Design review of the part built by this model. Coordinates are the model's own, in mm. Give positions to 0.01 mm unless a question says otherwise; leave off trailing zeros. Write each loop counter-clockwise with the first axis right and the second up, starting at its lowest first coordinate (ties: lowest second). Pieces come first, ordered by that corner, then holes. Notation, with made-up numbers: M 42,18 L 59,18 A6 ccw 59,26 Z; hole C 26.5,-18.5 d1. An arc over 180 degrees is marked long. Use one line per item in the form item = value. Start each with the question number.
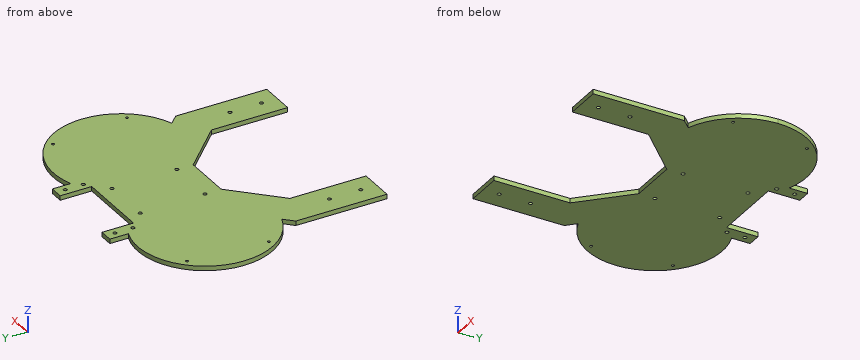
from build123d import *

# Parameters (mm, degrees)
SKETCH1_R           = 2
BOSS_EXTRUDE1_DEPTH = 5
SKETCH2_R           = 2
BOSS_EXTRUDE2_DEPTH = 5
BOSS_EXTRUDE3_START = -5
SKETCH3_R           = 1.4732
SKETCH3_R_2         = 2
BOSS_EXTRUDE3_DEPTH = 5


with BuildPart() as part:
    # Sketch1 → Boss-Extrude1 (new body)
    with BuildSketch(Plane.XY):
        Polygon((-40, 70), (-55, 70), (-55, -70), (55, -70), (55, 70), (40, 70), (40, 35), (-40, 35), align=None)
        with Locations((-27, -52)):
            Circle(SKETCH1_R, mode=Mode.SUBTRACT)
        with Locations((27, -52)):
            Circle(SKETCH1_R, mode=Mode.SUBTRACT)
        with Locations((-27, 20)):
            Circle(SKETCH1_R, mode=Mode.SUBTRACT)
        with Locations((-47.5, 40)):
            Circle(SKETCH1_R, mode=Mode.SUBTRACT)
        with Locations((-47.5, 60)):
            Circle(SKETCH1_R, mode=Mode.SUBTRACT)
        with Locations((27, 20)):
            Circle(SKETCH1_R, mode=Mode.SUBTRACT)
        with Locations((47.5, 40)):
            Circle(SKETCH1_R, mode=Mode.SUBTRACT)
        with Locations((47.5, 60)):
            Circle(SKETCH1_R, mode=Mode.SUBTRACT)
    extrude(amount=BOSS_EXTRUDE1_DEPTH)

    # Sketch2 → Boss-Extrude2 (add)
    with BuildSketch(Plane.XY):
        Polygon((-26.715726767, -70), (-55, -41.715726767), (-115, -101.715728753), (-115, -203), (-75, -203), (-75, -118.284271635), align=None)
        with Locations((-95, -185.5)):
            Circle(SKETCH2_R, mode=Mode.SUBTRACT)
        with Locations((-95, -150.5)):
            Circle(SKETCH2_R, mode=Mode.SUBTRACT)
    boss_extrude2 = extrude(amount=BOSS_EXTRUDE2_DEPTH)

    # Mirror1: Boss-Extrude2 across plane
    add(boss_extrude2.mirror(Plane(origin=(0, 0, 0), x_dir=(0, 0, 1), z_dir=(1, 0, 0))))

    # Sketch3 → Boss-Extrude3 (add)
    # profile 1 of 4: a face of its own
    with BuildSketch(Plane.XY.offset(5).offset(BOSS_EXTRUDE3_START)):
        with BuildLine():
            ThreePointArc((-55, 49.531907673), (-151.188193929, 4.063504127), (-105.126050476, -91.841778902))
            Line((-105.126050476, -91.841778902), (-55, -41.715726767))
            Line((-55, -41.715726767), (-55, 49.531907673))
        make_face()
        with Locations((-135.79276299, -59.716409454)):
            Circle(SKETCH3_R, mode=Mode.SUBTRACT)
        with Locations((-128.22970773, 26.72970773)):
            Circle(SKETCH3_R, mode=Mode.SUBTRACT)
    # profile 2 of 4: a face of its own
    with BuildSketch(Plane.XY.offset(5).offset(BOSS_EXTRUDE3_START)):
        with BuildLine():
            ThreePointArc((-105.126050476, -91.841778902), (-72.958779258, -95.619903442), (-42.197872056, -85.482144776))
            Line((-42.197872056, -85.482144776), (-26.715726767, -70))
            Line((-26.715726767, -70), (-23.719721734, -70))
            ThreePointArc((-23.719721734, -70), (-10.202344029, -47.138851639), (-5.5, -21))
            ThreePointArc((-5.5, -21), (-12.064844908, 9.685982916), (-30.610121267, 35))
            Line((-30.610121267, 35), (-40, 35))
            Line((-40, 35), (-40, 42.124876238))
            ThreePointArc((-40, 42.124876238), (-47.292831667, 46.247929123), (-55, 49.531907673))
            Line((-55, 49.531907673), (-55, -41.715726767))
            Line((-55, -41.715726767), (-105.126050476, -91.841778902))
        make_face()
        with Locations((-27, -52)):
            Circle(SKETCH3_R_2, mode=Mode.SUBTRACT)
        with Locations((-27, 20)):
            Circle(SKETCH3_R_2, mode=Mode.SUBTRACT)
        with Locations((-47.5, 40)):
            Circle(SKETCH3_R_2, mode=Mode.SUBTRACT)
    # profile 3 of 4: a face of its own
    with BuildSketch(Plane.XY.offset(5).offset(BOSS_EXTRUDE3_START)):
        with BuildLine():
            ThreePointArc((30.610121267, 35), (5.660968749, -16.088849276), (23.719721734, -70))
            Line((23.719721734, -70), (26.715726767, -70))
            Line((26.715726767, -70), (42.197872056, -85.482144776))
            ThreePointArc((42.197872056, -85.482144776), (72.958779258, -95.619903442), (105.126050476, -91.841778902))
            Line((105.126050476, -91.841778902), (55, -41.715726767))
            Line((55, -41.715726767), (55, 49.531907673))
            ThreePointArc((55, 49.531907673), (47.292831667, 46.247929123), (40, 42.124876238))
            Line((40, 42.124876238), (40, 35))
            Line((40, 35), (30.610121267, 35))
        make_face()
        with Locations((27, -52)):
            Circle(SKETCH3_R_2, mode=Mode.SUBTRACT)
        with Locations((27, 20)):
            Circle(SKETCH3_R_2, mode=Mode.SUBTRACT)
        with Locations((47.5, 40)):
            Circle(SKETCH3_R_2, mode=Mode.SUBTRACT)
    # profile 4 of 4: a face of its own
    with BuildSketch(Plane.XY.offset(5).offset(BOSS_EXTRUDE3_START)):
        with BuildLine():
            Line((55, -41.715726767), (105.126050476, -91.841778902))
            ThreePointArc((105.126050476, -91.841778902), (141.622638137, -64.462893451), (155.5, -21))
            ThreePointArc((155.5, -21), (123.584219849, 40.390145789), (55, 49.531907673))
            Line((55, 49.531907673), (55, -41.715726767))
        make_face()
        with Locations((135.79276299, -59.716409454)):
            Circle(SKETCH3_R, mode=Mode.SUBTRACT)
        with Locations((128.22970773, 26.72970773)):
            Circle(SKETCH3_R, mode=Mode.SUBTRACT)
    extrude(amount=BOSS_EXTRUDE3_DEPTH)


solid = part.part
1. We need section C-C (x = 15). State the section outline as (y, z) points, and give its area (3 significant figures).
2. Clearance check with flat-ended pins moving along their axes: pin 1 Ø1 at (y, z) = (38, 4) entering from +X; pin 2 Ø6.5 at (x, y) = (47.5, 40) entering from +Z; pin 3 Ø2.5 at (x, y) = (-95, -185.5) entering from +Z; pin 4 Ø2 at (y, z) = (-86.5, 4) entering from +X. State where each tip first meets the part, or that it passes through.
3. We need section A-A (y = -176). State the section outline as (x, z) points.
4. We need section B-B (y = -81.5). State the section outline as (x, z) points, and give its area (3 significant figures).
5. We need section D-D (z = 2.1). Give the number of separate pieces and of enclosed holes in the cut face, and give its area (3 significant figures).
6. To check wall thickness, follow L1, parallel to X at y = -153.5, z = 1.5; L2, parallel to Y at x = 27, z = 2.7; L3, parallel to Y at x = 47.5, z = 1.65. State the ranges of each line that lie inside material, in increasing order.
Answer block:
q1.outline = M -70,0 L 35,0 L 35,5 L -70,5 Z
q1.area = 525 mm^2
q2.pin_1 = 127.43
q2.pin_2 = 5
q2.pin_3 = through
q2.pin_4 = 118.77
q3.outline = M -115,0 L -75,0 L -75,5 L -115,5 Z; M 75,0 L 115,0 L 115,5 L 75,5 Z
q4.outline = M -124.83,0 L -38.22,0 L -38.22,5 L -124.83,5 Z; M 38.22,0 L 124.83,0 L 124.83,5 L 38.22,5 Z
q4.area = 866 mm^2
q5.separate_pieces = 1
q5.enclosed_holes = 16
q5.area = 47,600 mm^2
q6.L1 = -115 to -75, 75 to 115
q6.L2 = -70.28 to -54, -50 to 18, 22 to 35
q6.L3 = -90.78 to 38, 42 to 58, 62 to 70
